Here's how the part is built. I have some questions about the finished solid (model axes, mm). A direction names the side the tool comes from. Round coordinates to 2 decimals unless told otherwise and drop trailing zeros. Loops run counter-clockwise (first coordinate to the right, second up) from the corner with the lowest first, then second, coordinate; pieces in that order, holes last. Notation, with made-up numbers: M 8.25,16 L 39.25,16 A18 ccw 39.25,41 Z; hole C 28,49.25 d5. An arc over 180 degrees is marked long. Use a Markdown table: item, result.
from build123d import *
from OCP.BRepFilletAPI import BRepFilletAPI_MakeChamfer

# Parameters (mm, degrees)
BOSS_EXTRUDE1_DEPTH      = 8.38
BOSS_EXTRUDE1_DEPTH_BACK = 3.18
SKETCH1_W                = 0.64
SKETCH1_H                = 0.64
SKETCH2_W                = 2.54
SKETCH2_H                = 2.34
BOSS_EXTRUDE2_DEPTH      = 2.54
CHAMFER1_SIZE            = 0.3
CHAMFER1_SIZE2           = 0.080384758


with BuildPart() as part:
    # Sketch1 → Boss-Extrude1 (new, two sides: drawn at the far end of the back side and taken through both)
    with BuildSketch(Plane(origin=(0, 0, 0), x_dir=(1, 0, 0), z_dir=(0, 1, 0)).offset(-BOSS_EXTRUDE1_DEPTH_BACK)):
        Rectangle(SKETCH1_W, SKETCH1_H)
    extrude(amount=BOSS_EXTRUDE1_DEPTH + BOSS_EXTRUDE1_DEPTH_BACK)

    # Sketch2 → Boss-Extrude2 (add)
    with BuildSketch(Plane(origin=(0, 0, 0), x_dir=(1, 0, 0), z_dir=(0, 1, 0))):
        Rectangle(SKETCH2_W, SKETCH2_H)
    extrude(amount=BOSS_EXTRUDE2_DEPTH)

    # Chamfer1: one chamfer whose edges measure the first distance from different faces: ONE call of the kernel's chamfer builder (chamfer() names one face for all edges)
    chamfer1_edges_1 = [part.edges().sort_by_distance(p)[0] for p in [
        (-0.32, 8.38, 0),
    ]]
    chamfer1_side_1 = [part.faces().sort_by_distance(p)[0] for p in [
        (-0.32, 5.46, 0),
    ]]
    chamfer1_edges_2 = [part.edges().sort_by_distance(p)[0] for p in [
        (0.32, -3.18, 0),
    ]]
    chamfer1_side_2 = [part.faces().sort_by_distance(p)[0] for p in [
        (0.32, -1.59, 0),
    ]]
    chamfer1_edges_3 = [part.edges().sort_by_distance(p)[0] for p in [
        (0, -3.18, 0.32),
    ]]
    chamfer1_side_3 = [part.faces().sort_by_distance(p)[0] for p in [
        (0, -1.59, 0.32),
    ]]
    chamfer1_edges_4 = [part.edges().sort_by_distance(p)[0] for p in [
        (-0.32, -3.18, 0),
    ]]
    chamfer1_side_4 = [part.faces().sort_by_distance(p)[0] for p in [
        (-0.32, -1.59, 0),
    ]]
    chamfer1_edges_5 = [part.edges().sort_by_distance(p)[0] for p in [
        (0, -3.18, -0.32),
    ]]
    chamfer1_side_5 = [part.faces().sort_by_distance(p)[0] for p in [
        (0, -1.59, -0.32),
    ]]
    chamfer1_edges_6 = [part.edges().sort_by_distance(p)[0] for p in [
        (0, 8.38, 0.32),
    ]]
    chamfer1_side_6 = [part.faces().sort_by_distance(p)[0] for p in [
        (0, 5.46, 0.32),
    ]]
    chamfer1_edges_7 = [part.edges().sort_by_distance(p)[0] for p in [
        (0.32, 8.38, 0),
    ]]
    chamfer1_side_7 = [part.faces().sort_by_distance(p)[0] for p in [
        (0.32, 5.46, 0),
    ]]
    chamfer1_edges_8 = [part.edges().sort_by_distance(p)[0] for p in [
        (0, 8.38, -0.32),
    ]]
    chamfer1_side_8 = [part.faces().sort_by_distance(p)[0] for p in [
        (0, 5.46, -0.32),
    ]]
    chamfer1 = BRepFilletAPI_MakeChamfer(part.part.solid().wrapped)
    for e in chamfer1_edges_1:
        chamfer1.Add(CHAMFER1_SIZE, CHAMFER1_SIZE2, e.wrapped, chamfer1_side_1[0].wrapped)  # the first distance lies on this face
    for e in chamfer1_edges_2:
        chamfer1.Add(CHAMFER1_SIZE, CHAMFER1_SIZE2, e.wrapped, chamfer1_side_2[0].wrapped)  # the first distance lies on this face
    for e in chamfer1_edges_3:
        chamfer1.Add(CHAMFER1_SIZE, CHAMFER1_SIZE2, e.wrapped, chamfer1_side_3[0].wrapped)  # the first distance lies on this face
    for e in chamfer1_edges_4:
        chamfer1.Add(CHAMFER1_SIZE, CHAMFER1_SIZE2, e.wrapped, chamfer1_side_4[0].wrapped)  # the first distance lies on this face
    for e in chamfer1_edges_5:
        chamfer1.Add(CHAMFER1_SIZE, CHAMFER1_SIZE2, e.wrapped, chamfer1_side_5[0].wrapped)  # the first distance lies on this face
    for e in chamfer1_edges_6:
        chamfer1.Add(CHAMFER1_SIZE, CHAMFER1_SIZE2, e.wrapped, chamfer1_side_6[0].wrapped)  # the first distance lies on this face
    for e in chamfer1_edges_7:
        chamfer1.Add(CHAMFER1_SIZE, CHAMFER1_SIZE2, e.wrapped, chamfer1_side_7[0].wrapped)  # the first distance lies on this face
    for e in chamfer1_edges_8:
        chamfer1.Add(CHAMFER1_SIZE, CHAMFER1_SIZE2, e.wrapped, chamfer1_side_8[0].wrapped)  # the first distance lies on this face
    add(Compound.cast(chamfer1.Shape()), mode=Mode.REPLACE)


solid = part.part
1. Imagine slicing it at A-A, the plane x = -0.1. Write out the boundary of the cut face in (y, z).
Answer sheet:
| item | result |
|---|---|
| outline | M -3.18,-0.24 L -2.88,-0.32 L 0,-0.32 L 0,-1.17 L 2.54,-1.17 L 2.54,-0.32 L 8.08,-0.32 L 8.38,-0.24 L 8.38,0.24 L 8.08,0.32 L 2.54,0.32 L 2.54,1.17 L 0,1.17 L 0,0.32 L -2.88,0.32 L -3.18,0.24 Z |
2. For pin 1 Ø0.7 at (y, z) = (-1, 0) entering from -X; pin 2 Ø1 at (y, z) = (5.5, -1) entering from +X; pin 3 Ø0.5 at (x, y) = (0, -1) entering from -Z, each with a flat end and sliding along its axis, tell me the tip position at first contact or that it passes through.
Answer sheet:
| item | result |
|---|---|
| pin 1 | x = -0.32 |
| pin 2 | through |
| pin 3 | z = -0.32 |
3. Which directions (+Z, -Z, +X, -X, +Y, -Y) give clear straight access to the entire face, cutting with the end or side of a thin tool? Please do faces 1 (the face through (0, 0, -1)), 2 (the face through (-1.27, 1, 0)).
Answer sheet:
| item | result |
|---|---|
| face 1 | -Y |
| face 2 | +Z, -Z, -X, +Y, -Y |
4. Imagine slicing it at B-B, the plane z = -0.1. Write out the boundary of the cut face in (x, y).
Answer sheet:
| item | result |
|---|---|
| outline | M -1.27,0 L -0.32,0 L -0.32,-2.88 L -0.24,-3.18 L 0.24,-3.18 L 0.32,-2.88 L 0.32,0 L 1.27,0 L 1.27,2.54 L 0.32,2.54 L 0.32,8.08 L 0.24,8.38 L -0.24,8.38 L -0.32,8.08 L -0.32,2.54 L -1.27,2.54 Z |
5. Imagine slicing it at C-C, the plane y = 5. Write out the boundary of the cut face in (x, z).
Answer sheet:
| item | result |
|---|---|
| outline | M -0.32,-0.32 L 0.32,-0.32 L 0.32,0.32 L -0.32,0.32 Z |
6. Imagine slicing it at D-D, the plane x = 1.1. Write out the boundary of the cut face in (y, z).
Answer sheet:
| item | result |
|---|---|
| outline | M 0,-1.17 L 2.54,-1.17 L 2.54,1.17 L 0,1.17 Z |
7. I need wall thicknesses on probe 1 along Y at (x, z) = (-0.9, -1); probe 2 along X at (y, z) = (-0.5, -0.05). Which ranges of each line are inside material? Lowest first, please. Write a range as from..to.
Answer sheet:
| item | result |
|---|---|
| probe 1 | 0..2.54 |
| probe 2 | -0.32..0.32 |
